Source: three-view drawing plus pictorial views. Frame: mm from the lowest corner of the part. A direction names the side the tool comes from. Give positions to 0.01 mm unless a question says otherwise; leave off trailing zeros. Loops run counter-clockwise (first coordinate to the right, second up) from the corner with the lowest first, then second, coordinate; pieces in that order, holes last. Notation, with made-up numbers: (67.25, -34.75) - (72.25, -34.75) arc R28 cw to (72.25, -3.75) - close; hole circle Ø2 at (56, 28). An arc over 180 degrees is marked (long way). Write each question's results on one line, items separated by ' | '. Start each with the question number.
(1) Cut plane D-D on z = 12.6. Return the cut outline in (x, y), then the cut area to 3 significant figures.
(2) Cut plane A-A on y = 5.25. Return the cut outline in (x, z), then the cut area to 3 significant figures.
(3) Pull-direction query (Z, two-part tool) for the marked faces 4, 5 and 6; classes: pulls with the +Z half, pulls with the -Z half, needs draft (parallel to the pull), parting line crosses it, or undercut.
(4) Cut plane B-B on x = 12.6. Return the cut outline in (y, z).
(5) Contact query for a flat-ended pin moving along its axis: pin 1 (1 mm diameter, centred on y = 16, z = 6, fed in from +X). Output: stop coordinate, or through.
(6) Material intervals for line 1 along X through (y, z) = (12.6, 1.9); line 2 along X through (y, z) = (23.3, 12.6); line 3 along Y through (x, z) = (37, 3.75), sorted ascending. Write a range as [from, to].
(7) Cut plane C-C on y = 12.6. Return the cut outline in (x, z), then the cut area to 3 significant figures.
(8) Reachability of the marked faces 1, 2 and 3 from +Z, -Z, +X, -X, +Y, -Y: full face, straight path, thin tool, end or side. Return the list, or none.
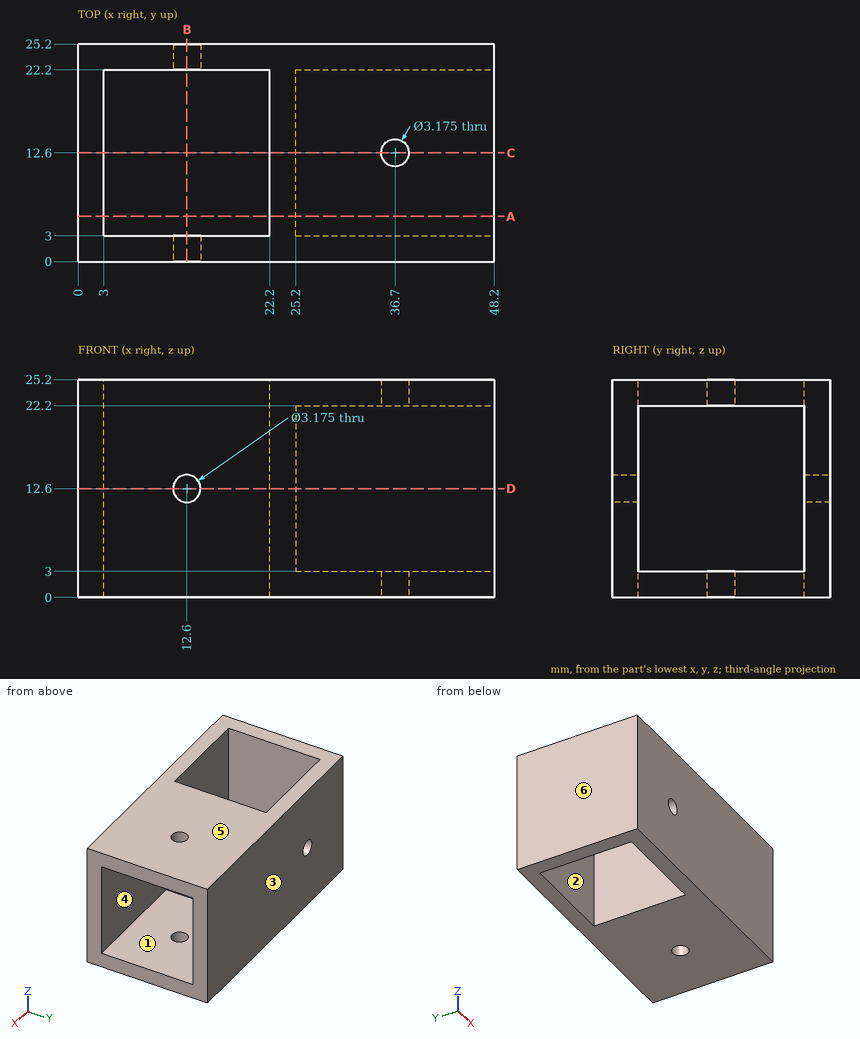
Ans:
1) outline: (0, 0) - (11.01, 0) - (11.01, 3) - (3, 3) - (3, 22.2) - (11.01, 22.2) - (11.01, 25.2) - (0, 25.2) - close; (14.19, 0) - (48.2, 0) - (48.2, 3) - (25.2, 3) - (25.2, 22.2) - (48.2, 22.2) - (48.2, 25.2) - (14.19, 25.2) - (14.19, 22.2) - (22.2, 22.2) - (22.2, 3) - (14.19, 3) - close | area: 385 mm^2
2) outline: (0, 0) - (3, 0) - (3, 25.2) - (0, 25.2) - close; (22.2, 0) - (48.2, 0) - (48.2, 3) - (25.2, 3) - (25.2, 22.2) - (48.2, 22.2) - (48.2, 25.2) - (22.2, 25.2) - close | area: 289 mm^2
3) face 4: undercut | face 5: pulls with the +Z half | face 6: needs draft
4) outline: (0, 0) - (3, 0) - (3, 11.01) - (0, 11.01) - close; (0, 14.19) - (3, 14.19) - (3, 25.2) - (0, 25.2) - close; (22.2, 0) - (25.2, 0) - (25.2, 11.01) - (22.2, 11.01) - close; (22.2, 14.19) - (25.2, 14.19) - (25.2, 25.2) - (22.2, 25.2) - close
5) pin 1: x = 25.2
6) line 1: [0, 3], [22.2, 35.11], [38.29, 48.2] | line 2: [0, 11.01], [14.19, 48.2] | line 3: [0, 3], [22.2, 25.2]
7) outline: (0, 0) - (3, 0) - (3, 25.2) - (0, 25.2) - close; (22.2, 0) - (35.11, 0) - (35.11, 3) - (25.2, 3) - (25.2, 22.2) - (35.11, 22.2) - (35.11, 25.2) - (22.2, 25.2) - close; (38.29, 0) - (48.2, 0) - (48.2, 3) - (38.29, 3) - close; (38.29, 22.2) - (48.2, 22.2) - (48.2, 25.2) - (38.29, 25.2) - close | area: 270 mm^2
8) face 1: +X | face 2: +Z, -Z | face 3: +Z, -Z, +X, -X, +Y
